The model under review builds one solid part; all positions refer to its coordinate system, in mm. Coordinates: 2 decimals unless noted, no trailing zeros. Write each loop counter-clockwise with the first axis right and the second up, starting at its lowest first coordinate (ties: lowest second). Pieces come first, ordered by that corner, then holes. Notation, with made-up numbers: M 10.5,-6.5 L 30.5,-6.5 A19 ccw 30.5,2.5 Z; hole C -2,72 d11. An arc over 180 degrees is marked long. Answer as a JSON object with one key per item and string values.
Autodesk Fusion 360 part; units mm, degrees
sketch "Skizze1" plane through (0, 0, 0) normal (0, 0, 1) x (1, 0, 0)
  line L0 (0, 0) -> (12, 0)
  line L1 (6, 0) -> (6, 11.5)
  line L2 (6, 11.5) -> (15, 11.5)
  line L3 (6, 11.5) -> (-3, 11.5)
  line L4 (-3, 11.5) -> (0, 0)
  line L5 (12, 0) -> (15, 11.5)
  line L6 (6, 11.5) -> (7.25, 11.5)
  line L7 (6, 11.5) -> (4.75, 11.5)
  line L8 (7.25, 11.5) -> (15, 11.5)
  line L9 (15, 11.5) -> (15, 61.5)
  line L10 (15, 61.5) -> (7.25, 61.5)
  line L11 (7.25, 61.5) -> (7.25, 11.5)
  line L12 (4.75, 11.5) -> (-3, 11.5)
  line L13 (-3, 11.5) -> (-3, 61.5)
  line L14 (-3, 61.5) -> (4.75, 61.5)
  line L15 (4.75, 61.5) -> (4.75, 11.5)
  dimension "d1" = 12
  dimension "d2" = 11.5
  dimension "d3" = 9
  dimension "d4" = 9
  dimension "d5" = 1.25
  dimension "d6" = 1.25
  dimension "d7" = 50
  dimension "d8" = 50
revolve "Drehen1" add sketch "Skizze1" angle 360 about axis through (6, 0, 0) along (0, 1, 0) contours L0 L1 L3 L4 L7 L12
extrude "Extrusion1" add sketch "Skizze1" along normal blind 9 contours L3 L12 L13 L14 L15 | L2 L8 L9 L10 L11
extrude "Extrusion2" add sketch "Skizze1" against normal blind 9 contours L3 L12 L13 L14 L15 | L2 L8 L9 L10 L11
chamfer "Fase1" distance 5 angle 45 6 edges at (-3, 61.5, 0) (-3, 36.5, 9) (-3, 36.5, -9) (15, 36.5, 9) (15, 36.5, -9) (15, 61.5, 0)
sketch "Skizze2" plane through (15, 0, 0) normal (1, 0, 0) x (0, 1, 0)
  line L0 (56.5, 4) -> (11.5, 4)
  line L1 (11.5, 4) -> (11.5, 0)
  line L2 (11.5, 0) -> (11.5, -4)
  line L3 (11.5, -4) -> (56.5, -4)
  line L4 (56.5, -4) -> (56.5, 4)
  line L5 (11.5, 0) -> (21.5, 0)
  line L6 (56.5, 0) -> (46.5, 0)
  dimension "d15" = 10
  dimension "d16" = 10
sketch "Skizze3" plane through (-3, 0, 0) normal (-1, 0, 0) x (0, -1, 0)
  line L0 (-56.5, -4) -> (-11.5, -4)
  line L1 (-11.5, -4) -> (-11.5, 0)
  line L2 (-11.5, 0) -> (-11.5, 4)
  line L3 (-11.5, 4) -> (-56.5, 4)
  line L4 (-56.5, 4) -> (-56.5, -4)
  line L5 (-11.5, 0) -> (-21.5, 0)
  line L6 (-56.5, 0) -> (-46.5, 0)
  line L7 (-48.1454, 2.85) -> (-49.7909, 0)
  line L8 (-49.7909, 0) -> (-48.1454, -2.85)
  line L9 (-48.1454, -2.85) -> (-44.8546, -2.85)
  line L10 (-44.8546, -2.85) -> (-43.2091, 0)
  line L11 (-43.2091, 0) -> (-44.8546, 2.85)
  line L12 (-44.8546, 2.85) -> (-48.1454, 2.85)
  line L13 (-23.1454, 2.85) -> (-24.7909, 0)
  line L14 (-24.7909, 0) -> (-23.1454, -2.85)
  line L15 (-23.1454, -2.85) -> (-19.8546, -2.85)
  line L16 (-19.8546, -2.85) -> (-18.2091, 0)
  line L17 (-18.2091, 0) -> (-19.8546, 2.85)
  line L18 (-19.8546, 2.85) -> (-23.1454, 2.85)
  point P0 (-56.5, 0)
  point P1 (-46.5, 0)
  point P2 (-21.5, 0)
  dimension "d17" = 10
  dimension "d18" = 10
  dimension "d29" = 2.85
  dimension "d30" = 2.85
hole "Bohrung1" at (15, 46.5, 0) direction (-1, 0, 0) diameter 3.6 depth 25 tip angle 180 counterbore diameter 6 counterbore depth 3.5
hole "Bohrung2" at (15, 21.5, 0) direction (-1, 0, 0) diameter 3.6 depth 25 tip angle 180 counterbore diameter 6 counterbore depth 3.5
extrude "Extrusion3" cut sketch "Skizze3" against normal blind 2.6 contours L13 L14 L15 L16 L17 L18 | L7 L8 L9 L10 L11 L12
chamfer "Fase2" distance 2 angle 45 8 edges at (8.625, 61.5, 9) (12.5, 59, 6.5) (12.5, 59, -6.5) (8.625, 61.5, -9) (-0.5, 59, -6.5) (3.375, 61.5, -9) (-0.5, 59, 6.5) (3.375, 61.5, 9)
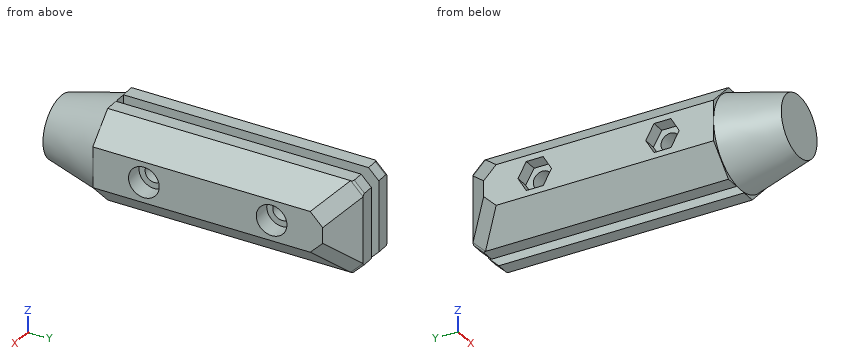
(1) For pin 1 Ø0.8 at (x, y) = (-2.5, 21.5) entering from -Z; pin 2 Ø4 at (y, z) = (21.5, 0) entering from +X; pin 3 Ø2.5 at (x, z) = (2, 5.5) entering from -Y; pin 4 Ø3 at (y, z) = (46.5, 0) entering from +X, all flat-tipped, find the tip position at first contact; note any pin that passes through.
Results list:
{"pin 1": "z = -4.9", "pin 2": "x = 11.5", "pin 3": "y = 0", "pin 4": "through"}
(2) Add section A-A on y = 17. Give the boundary of the cut face in (x, z), and give its area (3 significant figures).
Results list:
{"outline": "M -3,-4 L 2,-9 L 4.75,-9 L 4.75,9 L 2,9 L -3,4 Z; M 7.25,-9 L 10,-9 L 15,-4 L 15,4 L 10,9 L 7.25,9 Z", "area": "229 mm²"}
(3) Add section C-C on x = 6. Give the boundary of the cut face in (y, z), and give its area (4 significant figures).
Results list:
{"outline": "M 0,-6 L 11.5,-9 L 11.5,9 L 0,6 Z", "area": "172.5 mm²"}
(4) Add section B-B on y = 46.5. Give the boundary of the cut face in (x, z), and give its area (3 significant figures).
Results list:
{"outline": "M -3,-4 L 2,-9 L 4.75,-9 L 4.75,-1.8 L -0.4,-1.8 L -0.4,-2.85 L -3,-2.85 Z; M -3,2.85 L -0.4,2.85 L -0.4,1.8 L 4.75,1.8 L 4.75,9 L 2,9 L -3,4 Z; M 7.25,-9 L 10,-9 L 15,-4 L 15,-3 L 11.5,-3 L 11.5,-1.8 L 7.25,-1.8 Z; M 7.25,1.8 L 11.5,1.8 L 11.5,3 L 15,3 L 15,4 L 10,9 L 7.25,9 Z", "area": "159 mm²"}
(5) Add section D-D on z = -0.75. Count the separate pieces of the cut face and the enclosed holes in it, and give its area (3 significant figures).
Results list:
{"separate pieces": "5", "enclosed holes": "0", "area": "790 mm²"}
(6) Wall thickness on line 1 along Y through (x, z) = (2.8, 0); line 2 along Z through (x, y) = (8.65, 46.5); line 3 along Y through (x, z) = (0.9, 0): over which ranges is each line inside the solid? List them lowest first. Write a range as from..to.
Results list:
{"line 1": "0..19.7, 23.3..44.7, 48.3..61.5", "line 2": "-9..-1.8, 1.8..9", "line 3": "0..19.7, 23.3..44.7, 48.3..60.4"}
